Model file for the job. Use its own axes, mm. A direction names the side the tool comes from. Give positions to 0.01 mm unless a question says otherwise; leave off trailing zeros. Loops run counter-clockwise (first coordinate to the right, second up) from the corner with the lowest first, then second, coordinate; pieces in that order, holes last. Notation, with made-up numbers: (63.25, 9.25) - (77.25, 9.25) arc R18 ccw to (77.25, 34.25) - close; hole circle Ø1 at (17.25, -7). An arc over 180 degrees is marked (long way). Answer as CSV lines item,"result". Start each with the question number.
Item 1: Pull direction Z, two halves, no side cores. Call faces 1 (the flat face through (0, -7, 30)), 2 (the flat face through (12, -7, 16.8)), 3 (the cylindrical face through (22.43, -7.4, 16.2)), 4 (the flat face through (23, -7, 12)): pulls with the +Z half, pulls with the -Z half, needs draft (parallel to the pull), parting line crosses it, or undercut.
Item 2: Pin check, flat tips, straight feed: pin 1 (2 mm diameter, centred on y = -2.5, z = 31, fed in from +X); pin 2 (4.5 mm diameter, centred on x = 14, y = -7, fed in from +Z); pin 3 (6 mm diameter, centred on x = 4.5, z = 37, fed in from -Y); pin 4 (12 mm diameter, centred on x = 11.5, z = 18, fed in from +Y). Stop position of each tip, or through.
Item 3: Saw through at D-D on z = 25. Give the cut face in (x, y).
Item 4: Saw through at B-B on y = -10.75. Give the cut face in (x, z), plus the area to 3 significant figures.
Item 5: Drill centre lines: L1, parallel to Z at x = 5.5, y = -9.75; L2, parallel to Z at x = 10.5, y = -2.5; L3, parallel to X at y = -13.5, z = 33. Where is each one in solid material? Low to high. Write a range as from..to.
Item 6: Saw through at A-A on x = 4. Give the cut face in (y, z).
Item 7: Tool access for faces 5 (the flat face through (8, -7, 43)), 6 (the flat face through (14, -7, 9.8)), 7 (the flat face through (0, -7, 46.1)): list every direction of +Z, -Z, +X, -X, +Y, -Y with a clear straight run to the whole face (end or side of a thin tool).
Item 8: Saw through at C-C on x = 18. Give the cut face in (y, z), plus the area to 3 significant figures.
from build123d import *

# Parameters (mm, degrees)
F1_DEPTH = 15


with BuildPart() as f1:
    # F0 (on Front) → F1 (new body)
    with BuildSketch(Plane.XZ):
        with BuildLine():
            Line((-6, 0), (0, 0))
            Line((0, 0), (21, 0))
            ThreePointArc((21, 0), (22.414214, 0.585786), (23, 2))
            Line((23, 2), (23, 7))
            Line((23, 7), (6, 7))
            Line((6, 7), (6, 9.8))
            Line((6, 9.8), (23, 9.8))
            Line((23, 9.8), (23, 14.8))
            ThreePointArc((23, 14.8), (22.414214, 16.214214), (21, 16.8))
            Line((21, 16.8), (2, 16.8))
            ThreePointArc((2, 16.8), (0.585786, 17.385786), (0, 18.8))
            Line((0, 18.8), (0, 29.8))
            Line((0, 29.8), (0, 36.8))
            Line((0, 36.8), (0, 41.1))
            Line((0, 41.1), (8, 41.1))
            Line((8, 41.1), (8, 44.1))
            ThreePointArc((8, 44.1), (7.414214, 45.514214), (6, 46.1))
            Line((6, 46.1), (0, 46.1))
            Line((0, 46.1), (-6, 46.1))
            ThreePointArc((-6, 46.1), (-7.414214, 45.514214), (-8, 44.1))
            Line((-8, 44.1), (-8, 2))
            ThreePointArc((-8, 2), (-7.414214, 0.585786), (-6, 0))
        make_face()
    extrude(amount=F1_DEPTH)


solid = f1.part
Responses:
1,face 1,"undercut"
1,face 2,"undercut"
1,face 3,"pulls with the +Z half"
1,face 4,"needs draft"
2,pin 1,"x = 0"
2,pin 2,"z = 16.8"
2,pin 3,"through"
2,pin 4,"y = 0"
3,outline,"(-8, -15) - (0, -15) - (0, 0) - (-8, 0) - close"
4,outline,"(-8, 2) arc R2 ccw to (-6, 0) - (21, 0) arc R2 ccw to (23, 2) - (23, 7) - (6, 7) - (6, 9.8) - (23, 9.8) - (23, 14.8) arc R2 ccw to (21, 16.8) - (2, 16.8) arc R2 cw to (0, 18.8) - (0, 41.1) - (8, 41.1) - (8, 44.1) arc R2 ccw to (6, 46.1) - (-6, 46.1) arc R2 ccw to (-8, 44.1) - close"
4,area,"744 mm2"
5,L1,"0..16.8, 41.1..46.1"
5,L2,"0..7, 9.8..16.8"
5,L3,"-8..0"
6,outline,"(-15, 0) - (0, 0) - (0, 16.8) - (-15, 16.8) - close; (-15, 41.1) - (0, 41.1) - (0, 46.1) - (-15, 46.1) - close"
7,face 5,"+Z, +X, +Y, -Y"
7,face 6,"+X, +Y, -Y"
7,face 7,"+Z, +X, -X, +Y, -Y"
8,outline,"(-15, 0) - (0, 0) - (0, 7) - (-15, 7) - close; (-15, 9.8) - (0, 9.8) - (0, 16.8) - (-15, 16.8) - close"
8,area,"210 mm2"
